Source: three-view drawing plus pictorial views. Frame: mm from the lowest corner of the part. A direction names the side the tool comes from. Give positions to 0.01 mm unless a question says otherwise; leave off trailing zeros. Order: outer loops, then holes, each group sorted by start corner. A loop starts at its lowest first (then second) coordinate and runs counter-clockwise, first axis right, second up. Notation, with made-up numbers: M -1,84.25 L 43,84.25 A29 ccw 43,116.25 Z; hole C 41.25,13.5 d1. An arc over 180 degrees is marked long. Use CSV: the item, a comma, the result in double quotes. Start each with the question number.
Item 1: Section query C-C on z = 5.5. Return loops of the section in (x, y).
Item 2: First-contact query: pin 1 (1 mm diameter, centred on x = 9.5, y = 47, fed in from +Z); pin 2 (2 mm diameter, centred on x = 8.5, y = 47.5, fed in from -Z). Flat tips, straight axial feed; report the tip coordinate or a pass-through.
Item 3: Ray query, probe 1 along Y at (x, z) = (11.5, 8.75). Return the intervals inside material, ascending. Write a range as from..to.
Item 4: Section query A-A on x = 8.5. Return loops of the section in (y, z), and give its area (3 significant figures).
Item 5: Section query B-B on z = 18.5. Return loops of the section in (x, y) (1 decimal), and give its area (3 significant figures).
Item 6: Access query for the marked faces 1 and 2. Directions: +Z, -Z, +X, -X, +Y, -Y. A direction counts if a zero-diameter tool reaches every point of the face in a straight line with its end or side. Return the directions, or none.
Item 7: Section query D-D on z = 10.5. Return loops of the section in (x, y), and give its area (3 significant figures).
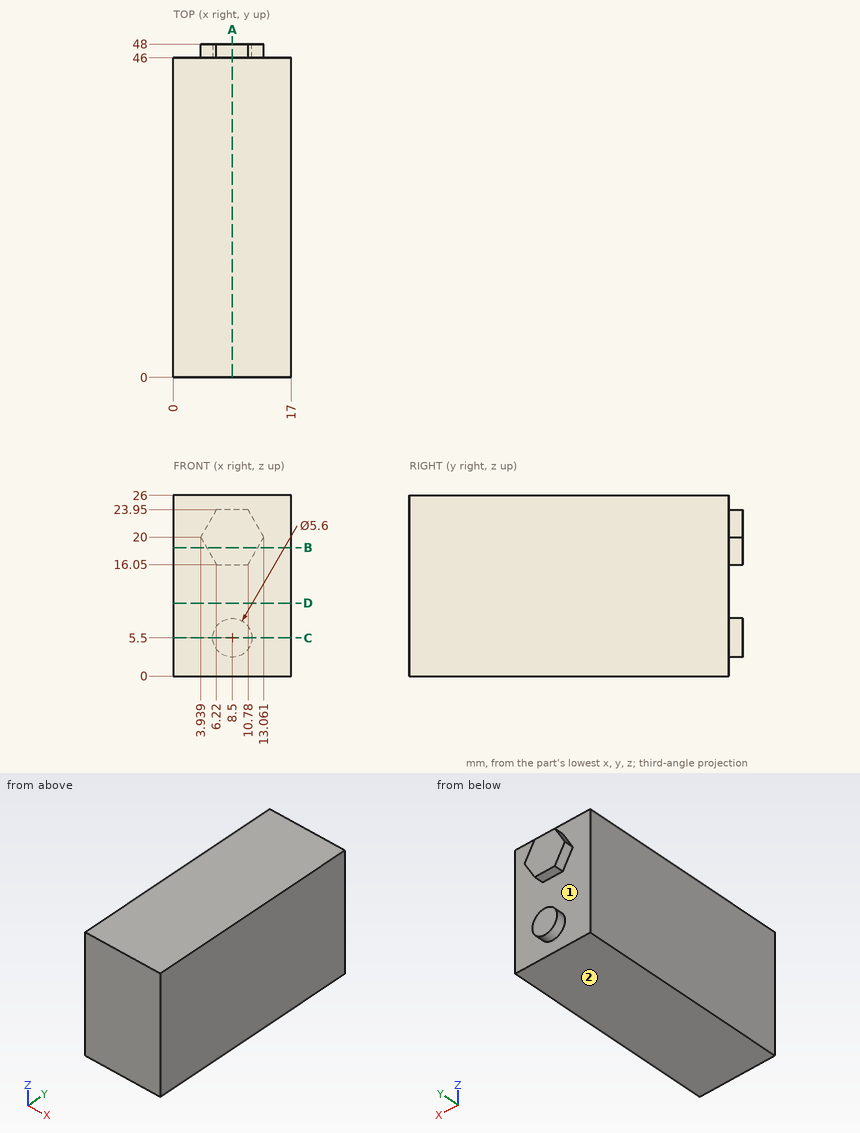
Verdict:
1,outline,"M 0,0 L 17,0 L 17,46 L 11.3,46 L 11.3,48 L 5.7,48 L 5.7,46 L 0,46 Z"
2,pin 1,"z = 23.95"
2,pin 2,"z = 2.7"
3,probe 1,"0..46"
4,outline,"M 0,0 L 46,0 L 46,2.7 L 48,2.7 L 48,8.3 L 46,8.3 L 46,16.05 L 48,16.05 L 48,23.95 L 46,23.95 L 46,26 L 0,26 Z"
4,area,"1,220 mm2"
5,outline,"M 0,0 L 17,0 L 17,46 L 12.2,46 L 12.2,48 L 4.8,48 L 4.8,46 L 0,46 Z"
5,area,"797 mm2"
6,face 1,"+Y"
6,face 2,"-Z, +X, -X, +Y, -Y"
7,outline,"M 0,0 L 17,0 L 17,46 L 0,46 Z"
7,area,"782 mm2"
